```python
from build123d import *

# Parameters (mm, degrees)
BOSS_EXTRUDE1_DEPTH = 2.5
FILLET1_R           = 3
FILLET2_R           = 1
FILLET3_R           = 2
SKETCH3_W           = 16.773949538
SKETCH3_H           = 15.481085324
BOSS_EXTRUDE2_DEPTH = 1
CHAMFER1_SIZE       = 0.5
SKETCH5_R           = 1.65
CUT_EXTRUDE3_DEPTH  = 45.453167491
SKETCH6_W           = 10
SKETCH6_H           = 10
CUT_EXTRUDE4_DEPTH  = 1
CHAMFER2_SIZE       = 0.25
CHAMFER3_SIZE       = 0.25
SKETCH7_W           = 4
SKETCH7_H           = 13.28
CUT_EXTRUDE5_DEPTH  = 45.408153531
CHAMFER4_SIZE       = 1
CUT_EXTRUDE6_DEPTH  = 0.25
CUT_EXTRUDE8_DEPTH  = 10
SKETCH11_W          = 19.67193657
SKETCH11_H          = 16.670050146
CUT_EXTRUDE9_DEPTH  = 0.25
CHAMFER5_SIZE       = 3
CHAMFER5_SIZE_2     = 0.262465991


# Some blends are built 0.0001 mm under size
with BuildPart() as part:
    # Sketch1 → Boss-Extrude1 (new body)
    with BuildSketch(Plane(origin=(0, 0, 0), x_dir=(1, 0, 0), z_dir=(0, 1, 0))):
        Polygon((0, -5.29), (0, 5.29), (-1, 6.29), (-1, 12.79), (9, 12.79), (11, 10.79), (31, 10.79), (33, 12.79), (42.5, 12.79), (42.5, 6.64), (26.5, 6.64), (26.5, -6.64), (42.5, -6.64), (42.5, -12.79), (33, -12.79), (31, -10.79), (11, -10.79), (9, -12.79), (-1, -12.79), (-1, -6.29), align=None)
    extrude(amount=BOSS_EXTRUDE1_DEPTH)

    # Fillet1
    fillet1_edges = [part.edges().sort_by_distance(p)[0] for p in [
        (-1, 1.25, -12.79),
        (42.5, 1.25, -12.79),
        (42.5, 1.25, 12.79),
        (-1, 1.25, 12.79),
    ]]
    fillet(fillet1_edges, radius=FILLET1_R)

    # Fillet2
    fillet2_edges = [part.edges().sort_by_distance(p)[0] for p in [
        (-1, 1.25, -6.29),
        (26.5, 1.25, -6.64),
        (26.5, 1.25, 6.64),
        (-1, 1.25, 6.29),
        (0, 1.25, 5.29),
        (0, 1.25, -5.29),
    ]]
    fillet(fillet2_edges, radius=FILLET2_R)

    # Fillet3
    fillet3_edges = [part.edges().sort_by_distance(p)[0] for p in [
        (9, 1.25, -12.79),
        (11, 1.25, -10.79),
        (31, 1.25, -10.79),
        (33, 1.25, -12.79),
        (33, 1.25, 12.79),
        (31, 1.25, 10.79),
        (11, 1.25, 10.79),
        (9, 1.25, 12.79),
    ]]
    fillet(fillet3_edges, radius=FILLET3_R)

    # Sketch3 → Boss-Extrude2 (add)
    with BuildSketch(Plane.XZ):
        with Locations((34.113025231, 0.175921424)):
            Rectangle(SKETCH3_W, SKETCH3_H)
    extrude(amount=-BOSS_EXTRUDE2_DEPTH)

    # Chamfer1
    chamfer1_edges = [part.edges().sort_by_distance(p)[0] for p in [
        (42.5, 1, 0),
        (42.5, 1.75, -6.64),
        (42.5, 1.75, 6.64),
    ]]
    chamfer(chamfer1_edges, length=CHAMFER1_SIZE)

    # Sketch5 → Cut-Extrude3 (cut, through all)
    with BuildSketch(Plane(origin=(0, 2.5, 0), x_dir=(1, 0, 0), z_dir=(0, 1, 0))):
        with Locations(Location((2, 9.79, 0), (0, 0, 270))):
            Circle(SKETCH5_R)
        with Locations(Location((2, -9.79, 0), (0, 0, 270))):
            Circle(SKETCH5_R)
        with Locations(Location((39.5, 9.79, 0), (0, 0, 270))):
            Circle(SKETCH5_R)
        with Locations(Location((39.5, -9.79, 0), (0, 0, 270))):
            Circle(SKETCH5_R)
    extrude(amount=-CUT_EXTRUDE3_DEPTH, mode=Mode.SUBTRACT)

    # Sketch6 → Cut-Extrude4 (cut)
    with BuildSketch(Plane(origin=(0, 2.5, 0), x_dir=(1, 0, 0), z_dir=(0, 1, 0))):
        with Locations((5.4, 0)):
            Rectangle(SKETCH6_W, SKETCH6_H)
    extrude(amount=-CUT_EXTRUDE4_DEPTH, mode=Mode.SUBTRACT)

    # Chamfer2
    chamfer2_edges = [part.edges().sort_by_distance(p)[0] for p in [
        (10.4, 2.5, 0),
        (5.4, 2.5, -5),
        (5.4, 2.5, 5),
    ]]
    chamfer(chamfer2_edges, length=CHAMFER2_SIZE)

    # Chamfer3
    chamfer3_edges = [part.edges().sort_by_distance(p)[0] for p in [
        (36.664213562, 0, 12.79),
        (5.085786438, 0, -12.79),
        (10, 0, -11.79),
        (21, 0, -10.79),
        (32, 0, -11.79),
        (32, 0, 11.79),
        (21, 0, 10.79),
        (10, 0, 11.79),
        (8.93693974, 0, -12.637759065),
        (33.06306026, 0, -12.637759065),
        (8.93693974, 0, 12.637759065),
        (33.06306026, 0, 12.637759065),
        (30.93693974, 0, 10.942240935),
        (11.06306026, 0, 10.942240935),
        (30.93693974, 0, -10.942240935),
        (11.06306026, 0, -10.942240935),
        (42.5, 0, 0),
        (-1, 0, -8.247106781),
        (36.664213562, 0, -12.79),
        (5.085786438, 0, 12.79),
        (-0.121320344, 0, 11.911320344),
        (41.621320344, 0, 11.911320344),
        (41.621320344, 0, -11.911320344),
        (-0.121320344, 0, -11.911320344),
        (-1, 0, 8.247106781),
        (-0.5, 0, 5.79),
        (0, 0, 0),
        (-0.5, 0, -5.79),
        (-0.923879533, 0, -6.32153013),
        (-0.923879533, 0, 6.32153013),
        (-0.076120467, 0, 5.25846987),
        (-0.076120467, 0, -5.25846987),
    ]]
    chamfer(chamfer3_edges, length=CHAMFER3_SIZE)

    # Sketch7 → Cut-Extrude5 (cut, through all)
    with BuildSketch(Plane(origin=(0, 1, 0), x_dir=(1, 0, 0), z_dir=(0, 1, 0))):
        with Locations((35, 0)):
            Rectangle(SKETCH7_W, SKETCH7_H)
    extrude(amount=-CUT_EXTRUDE5_DEPTH, mode=Mode.SUBTRACT)

    # Chamfer4
    chamfer4_edges = [part.edges().sort_by_distance(p)[0] for p in [
        (0.4, 1.5, 0),
    ]]
    chamfer(chamfer4_edges, length=CHAMFER4_SIZE - 0.0001)  # a hair under: the kernel refuses the full size

    # Sketch8 → Cut-Extrude6 (cut)
    with BuildSketch(Plane(origin=(0, 2.5, 0), x_dir=(1, 0, 0), z_dir=(0, 1, 0))):
        with BuildLine():
            Line((41.25, -9.79), (41.25, -7.89))
            Line((41.25, -7.89), (27.5, -7.89))
            ThreePointArc((27.5, -7.89), (25.909009742, -7.230990258), (25.25, -5.64))
            Line((25.25, -5.64), (25.25, 5.64))
            ThreePointArc((25.25, 5.64), (25.909009742, 7.230990258), (27.5, 7.89))
            Line((27.5, 7.89), (41.25, 7.89))
            Line((41.25, 7.89), (41.25, 9.79))
            ThreePointArc((41.25, 9.79), (40.737436867, 11.027436867), (39.5, 11.54))
            Line((39.5, 11.54), (33.828427125, 11.54))
            ThreePointArc((33.828427125, 11.54), (33.54141455, 11.482909649), (33.298097039, 11.320330086))
            Line((33.298097039, 11.320330086), (32.469669914, 10.491902961))
            ThreePointArc((32.469669914, 10.491902961), (31.41529403, 9.787391519), (30.171572875, 9.54))
            Line((30.171572875, 9.54), (11.828427125, 9.54))
            ThreePointArc((11.828427125, 9.54), (10.58470597, 9.787391519), (9.530330086, 10.491902961))
            Line((9.530330086, 10.491902961), (8.701902961, 11.320330086))
            ThreePointArc((8.701902961, 11.320330086), (8.45858545, 11.482909649), (8.171572875, 11.54))
            Line((8.171572875, 11.54), (2, 11.54))
            ThreePointArc((2, 11.54), (0.762563133, 11.027436867), (0.25, 9.79))
            Line((0.25, 9.79), (0.25, 6.807766953))
            Line((0.25, 6.807766953), (0.590990258, 6.466776695))
            ThreePointArc((0.590990258, 6.466776695), (1.078728948, 5.73682416), (1.25, 4.875786438))
            Line((1.25, 4.875786438), (1.25, -4.875786438))
            ThreePointArc((1.25, -4.875786438), (1.078728948, -5.73682416), (0.590990258, -6.466776695))
            Line((0.590990258, -6.466776695), (0.25, -6.807766953))
            Line((0.25, -6.807766953), (0.25, -9.79))
            ThreePointArc((0.25, -9.79), (0.762563133, -11.027436867), (2, -11.54))
            Line((2, -11.54), (8.171572875, -11.54))
            ThreePointArc((8.171572875, -11.54), (8.45858545, -11.482909649), (8.701902961, -11.320330086))
            Line((8.701902961, -11.320330086), (9.530330086, -10.491902961))
            ThreePointArc((9.530330086, -10.491902961), (10.58470597, -9.787391519), (11.828427125, -9.54))
            Line((11.828427125, -9.54), (30.171572875, -9.54))
            ThreePointArc((30.171572875, -9.54), (31.41529403, -9.787391519), (32.469669914, -10.491902961))
            Line((32.469669914, -10.491902961), (33.298097039, -11.320330086))
            ThreePointArc((33.298097039, -11.320330086), (33.54141455, -11.482909649), (33.828427125, -11.54))
            Line((33.828427125, -11.54), (39.5, -11.54))
            ThreePointArc((39.5, -11.54), (40.737436867, -11.027436867), (41.25, -9.79))
        make_face()
    extrude(amount=-CUT_EXTRUDE6_DEPTH, mode=Mode.SUBTRACT)

    # Sketch10 → Cut-Extrude8 (cut)
    with BuildSketch(Plane(origin=(0, 1, 0), x_dir=(1, 0, 0), z_dir=(0, 1, 0))):
        with BuildLine():
            Line((27.5, -6.64), (33, -6.64))
            Line((33, -6.64), (33, 6.64))
            Line((33, 6.64), (27.5, 6.64))
            ThreePointArc((27.5, 6.64), (26.792893219, 6.347106781), (26.5, 5.64))
            Line((26.5, 5.64), (26.5, -5.64))
            ThreePointArc((26.5, -5.64), (26.792893219, -6.347106781), (27.5, -6.64))
        make_face()
    extrude(amount=-CUT_EXTRUDE8_DEPTH, mode=Mode.SUBTRACT)

    # Sketch11 → Cut-Extrude9 (cut)
    with BuildSketch(Plane(origin=(0, 2.5, 0), x_dir=(1, 0, 0), z_dir=(0, 1, 0))):
        with Locations((26.029913711, 0)):
            Rectangle(SKETCH11_W, SKETCH11_H)
    extrude(amount=-CUT_EXTRUDE9_DEPTH, mode=Mode.SUBTRACT)

    # Chamfer5
    # the kernel refuses this chamfer: 3, 0.262465991 mm, written as the material it takes off along each edge
    with BuildSketch(Plane(origin=(35.865881996, 2.5, 15.68890224), x_dir=(0.9999943799678764, 0.0033526157940331697, 0), z_dir=(0, 0, -1))) as chamfer5_piece_1_section:
        Polygon((CHAMFER5_SIZE * 0.999994379968, CHAMFER5_SIZE * 0.00335261579403), (-CHAMFER5_SIZE_2 * 0.00335261578864, CHAMFER5_SIZE_2 * 0.999994378359), (0, 0), align=None)
    chamfer5_piece_1 = extrude(amount=16.847804479, mode=Mode.PRIVATE)
    chamfer5_piece_1 = split(chamfer5_piece_1, bisect_by=Plane(origin=(36.868035548, 2.25, 7.265), z_dir=(0, 1, 0)), keep=Keep.TOP, mode=Mode.PRIVATE)
    chamfer5_piece_1 = split(chamfer5_piece_1, bisect_by=Plane(origin=(36.868035548, 2.412888159, 11.54), z_dir=(0, 0, -1)), keep=Keep.TOP, mode=Mode.PRIVATE)
    add(chamfer5_piece_1, mode=Mode.SUBTRACT)
    with BuildSketch(Plane(origin=(35.865881996, 2.5, 1.15890224), x_dir=(0.9999943799678764, 0.0033526157940331697, 0), z_dir=(0, 0, -1))) as chamfer5_piece_2_section:
        Polygon((CHAMFER5_SIZE * 0.999994379968, CHAMFER5_SIZE * 0.00335261579403), (-CHAMFER5_SIZE_2 * 0.00335261578864, CHAMFER5_SIZE_2 * 0.999994378359), (0, 0), align=None)
    chamfer5_piece_2 = extrude(amount=9.04890224, mode=Mode.PRIVATE)
    chamfer5_piece_2 = split(chamfer5_piece_2, bisect_by=Plane(origin=(36.868035548, 2.25, -7.265), z_dir=(0, 1, 0)), keep=Keep.TOP, mode=Mode.PRIVATE)
    add(chamfer5_piece_2, mode=Mode.SUBTRACT)


solid = part.part
```
Verification items for the finished model (mm, model axes). A direction names the side the tool comes from. Give positions to 0.01 mm unless a question says otherwise; leave off trailing zeros. Loops run counter-clockwise (first coordinate to the right, second up) from the corner with the lowest first, then second, coordinate; pieces in that order, holes last.
1. Go/stop test with flat-tipped pins: pin 1 Ø1 at (x, z) = (37.5, -10) entering from -Y; pin 2 Ø10 at (x, z) = (6.5, -2) entering from +Y; pin 3 Ø0.5 at (y, z) = (0.5, -2.5) entering from -X; pin 4 Ø0.7 at (x, y) = (18, 1.5) entering from -Z. Record where each tip stops, or that it passes through.
2. Set-up check for faces 5 (the flat face through (9.99, 1.36, -11.8)), 6 (the flat face through (35, 1, -6.64)), 7 (the cylindrical face through (33.053, 1.391, 12.634)), 8 (the conical face through (30.995, 0.127, 10.833)): record each of +Z, -Z, +X, -X, +Y, -Y from which the full face is reachable in a straight line by a thin tool's end or side.
3. Section check B-B, the plane x = 6. Enter the section's corners in (y, z).
4. Mould release check, pull along X, two halves, no side actions. Record for faces 1 (the cylindrical face through (26.785, 1.141, 6.339)), 2 (the cylindrical face through (33.053, 1.391, -12.634)), 3 (the conical face through (41.56, 0.13, 11.8)), 4 (the flat face through (-1, 1, -8)): released by +X, released by -X, zero draft, split by the parting line, or undercut.
5. Thickness scan on line 1 (X direction, y = 0.85, z = 9.79); line 2 (X direction, y = 0.35, z = 3); line 3 (Y direction, x = 20.5, z = -6). Record the ranges inside material, lowest first.
Geometry says:
1. pin 1: stops at y = 0
1. pin 2: stops at y = 2.25
1. pin 3: stops at x = 0
1. pin 4: stops at z = -10.79
2. face 5: -Z, +Y, -Y
2. face 6: +Y
2. face 7: +Z, +Y, -Y
2. face 8: +Z, -Y
3. outline: (0, -12.54) - (0.25, -12.79) - (2.5, -12.79) - (2.5, -11.54) - (2.25, -11.54) - (2.25, -5) - (1.5, -5) - (1.5, 5) - (2.25, 5) - (2.25, 11.54) - (2.5, 11.54) - (2.5, 12.79) - (0.25, 12.79) - (0, 12.54) - close
4. face 1: undercut
4. face 2: undercut
4. face 3: released by +X
4. face 4: released by -X
5. line 1: x = -1 to 0.35, 3.65 to 37.85, 41.15 to 42.5
5. line 2: x = 0 to 26.5, 37 to 42.5
5. line 3: y = 0 to 2.25
